For this review, use the dimensioned drawing (mm, ordinates from the lowest corner) and the shaded views. A direction names the side the tool comes from. Give positions to 0.01 mm unless a question says otherwise; leave off trailing zeros. Write each loop counter-clockwise with the first axis right and the second up, starting at its lowest first coordinate (ties: lowest second). Pieces come first, ordered by that corner, then holes.
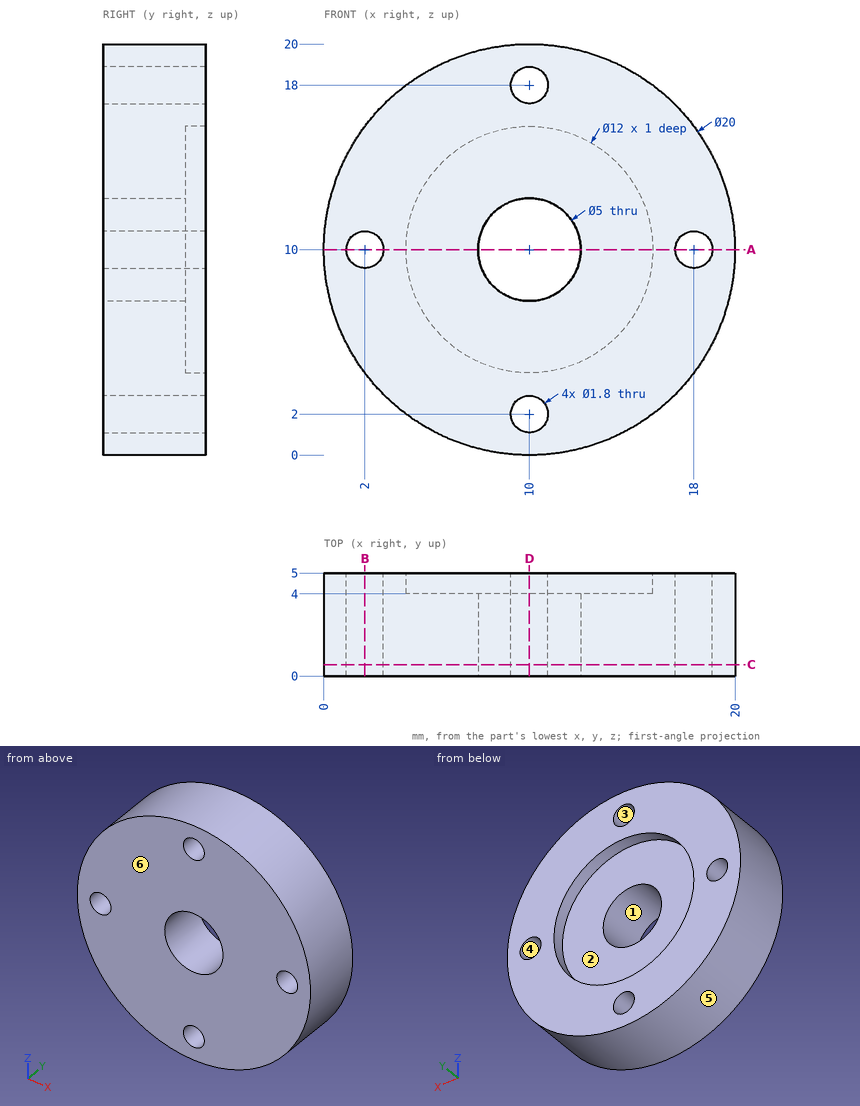
(1) We need section D-D (x = 10). Write out the cut boundary in (y, z).
(2) We need section A-A (z = 10). Write out the cut boundary in (x, y).
(3) We need section C-C (y = 0.55). Write out the cut boundary in (x, z).
(4) Clearance check with flat-ended pins moving along their axes: pin 1 Ø6 at (x, z) = (11.5, 11) entering from +Y; pin 2 Ø3 at (x, y) = (2, 2) entering from -Z; pin 3 Ø2 at (x, y) = (12.5, 4) entering from -Z. State where each tip first meets the part, or that it passes through.
(5) The part is to be moulded in two halves that separate along Z. For the marked faces 3, 4, 5 and 6, say which applies: +Z half, -Z half, draft (parallel to the pull), parting line (faces both ways), or undercut.
(6) We need section B-B (x = 2). Write out the cut boundary in (y, z).
(7) Tool access review of the marked faces 1 and 2: name each direction out of +Z, -Z, +X, -X, +Y, -Y from which nothing blocks a thin tool from reaching the whole face with its end or side.
(8) For L1, parallel to X at y = 1.8, z = 10; L2, parallel to X at y = 4.5, z = 10; L3, parallel to Z at x = 9.25, y = 2.4, list the stretches that pass through material, from the lowest coordinate up.
The answers:
1. outline: (0, 0) - (5, 0) - (5, 1.1) - (0, 1.1) - close; (0, 2.9) - (5, 2.9) - (5, 4) - (4, 4) - (4, 7.5) - (0, 7.5) - close; (0, 12.5) - (4, 12.5) - (4, 16) - (5, 16) - (5, 17.1) - (0, 17.1) - close; (0, 18.9) - (5, 18.9) - (5, 20) - (0, 20) - close
2. outline: (0, 0) - (1.1, 0) - (1.1, 5) - (0, 5) - close; (2.9, 0) - (7.5, 0) - (7.5, 4) - (4, 4) - (4, 5) - (2.9, 5) - close; (12.5, 0) - (17.1, 0) - (17.1, 5) - (16, 5) - (16, 4) - (12.5, 4) - close; (18.9, 0) - (20, 0) - (20, 5) - (18.9, 5) - close
3. outline: circle Ø20 at (10, 10); hole circle Ø1.8 at (2, 10); hole circle Ø5 at (10, 10); hole circle Ø1.8 at (10, 2); hole circle Ø1.8 at (10, 18); hole circle Ø1.8 at (18, 10)
4. pin 1: stops at y = 4
4. pin 2: stops at z = 2.4
4. pin 3: stops at z = 0.11
5. face 3: undercut
5. face 4: undercut
5. face 5: parting line
5. face 6: draft
6. outline: (0, 4) - (5, 4) - (5, 9.1) - (0, 9.1) - close; (0, 10.9) - (5, 10.9) - (5, 16) - (0, 16) - close
7. face 1: +Y, -Y
7. face 2: +Y
8. L1: x = 0 to 1.1, 2.9 to 7.5, 12.5 to 17.1, 18.9 to 20
8. L2: x = 0 to 1.1, 2.9 to 4, 16 to 17.1, 18.9 to 20
8. L3: z = 0.03 to 1.5, 2.5 to 7.62, 12.38 to 17.5, 18.5 to 19.97
